CAD build for the part. Positions are in the model's coordinates, mm. A direction names the side the tool comes from. Coordinates: 2 decimals unless noted, no trailing zeros. Write each loop counter-clockwise with the first axis right and the second up, starting at its lowest first coordinate (ties: lowest second). Pieces come first, ordered by that corner, then holes. Notation, with made-up numbers: (-37, -10) -> (-5, -10) arc R7 cw to (-5, 1) -> close; hole circle Ø7 at (38.25, 51). An arc over 180 degrees is marked (long way). Answer as CSV lines item,"result".
```python
from build123d import *

# Parameters (mm, degrees)
DOME1_FACE_RADIUS       = 12.7
DOME1_HEIGHT            = 3.81
CUT_EXTRUDE1_DEPTH      = 53.685870022
CUT_EXTRUDE1_DEPTH_BACK = 53.685870022


with BuildPart() as part:
    # Sketch1 → Revolve2 (revolve)
    with BuildSketch(Plane.XY, mode=Mode.PRIVATE) as revolve2_sk:
        Polygon((0, 0), (0, 45.72), (-12.7, 45.72), (-12.7, 43.18), (-6.35, 43.18), (-6.35, 0), (-0.453180755, 0), align=None)
    revolve(revolve2_sk.sketch.rotate(Axis((0, 0, 0), (0, 1, 0)), 270), axis=Axis((0, 0, 0), (0, 1, 0)))

    # Dome1: a dome of height H over a round flat face of radius A is a cap of a sphere of radius (A * A + H * H) / (2 * H)
    dome1_r = (DOME1_FACE_RADIUS * DOME1_FACE_RADIUS + DOME1_HEIGHT * DOME1_HEIGHT) / (2 * DOME1_HEIGHT)
    dome1_base = Plane((0, 45.72, 0), z_dir=(0, 1, 0))
    with Locations(dome1_base.offset(DOME1_HEIGHT - dome1_r)):
        dome1_ball = Sphere(dome1_r, mode=Mode.PRIVATE)
    add(split(dome1_ball, bisect_by=dome1_base, keep=Keep.TOP, mode=Mode.PRIVATE))

    # Sketch2 → Cut-Extrude1 (cut, two sides: drawn at the far end of the back side and taken through both)
    with BuildSketch(Plane.XY.offset(-CUT_EXTRUDE1_DEPTH_BACK)):
        Polygon((7.09988746, 57.306992364), (-7.09988746, 57.306992364), (-2.413050327, 47.453982482), (2.413050327, 47.453982482), align=None)
    extrude(amount=CUT_EXTRUDE1_DEPTH + CUT_EXTRUDE1_DEPTH_BACK, mode=Mode.SUBTRACT)


solid = part.part
```
Item 1: Saw through at C-C on y = 22. Give the cut face in (x, z).
Answer below:
outline,"circle Ø12.7 at (0, 0)"
Item 2: Saw through at B-B on x = 0. Give the cut face in (y, z).
Answer below:
outline,"(0, -6.35) -> (43.18, -6.35) -> (43.18, -12.7) -> (45.72, -12.7) arc R23.07 ccw to (47.45, -9.56) -> (47.45, 9.56) arc R23.07 ccw to (45.72, 12.7) -> (43.18, 12.7) -> (43.18, 6.35) -> (0, 6.35) -> close"
Item 3: Saw through at A-A on z = 0. Give the cut face in (x, y), and give its area (3 significant figures).
Answer below:
outline,"(-12.7, 43.18) -> (-6.35, 43.18) -> (-6.35, 0) -> (6.35, 0) -> (6.35, 43.18) -> (12.7, 43.18) -> (12.7, 45.72) arc R23.07 ccw to (3.29, 49.29) -> (2.41, 47.45) -> (-2.41, 47.45) -> (-3.29, 49.29) arc R23.07 ccw to (-12.7, 45.72) -> close"
area,"667 mm2"
Item 4: Two-plate mould, pull along X, no slides. Class faces 4 (the flat face through (2.75, 48.16, -0.13)), 5 (the cylindrical face through (7.7, 44.4, 10.1)), 6 (the flat face through (-6, 43.18, -3)): pulls with the +X half, pulls with the -X half, needs draft (parallel to the pull), parting line crosses it, or undercut.
Answer below:
face 4,"undercut"
face 5,"parting line crosses it"
face 6,"needs draft"
Item 5: Saw through at D-D on z = 7.75. Give the cut face in (x, y), and give its area (3 significant figures).
Answer below:
outline,"(-10.06, 43.18) -> (10.06, 43.18) -> (10.06, 45.72) arc R21.73 ccw to (2.68, 48.02) -> (2.41, 47.45) -> (-2.41, 47.45) -> (-2.68, 48.02) arc R21.73 ccw to (-10.06, 45.72) -> close"
area,"81.1 mm2"
Item 6: Wall check: line 1 (Y direction, x = 2.25, z = -8.25); line 2 (Y direction, x = -1.75, z = 5.5); line 3 (X direction, y = 44, z = 0). Give the ranges that are in metal, low to high. Write a range as from..to.
Answer below:
line 1,"y = 43.18..47.45"
line 2,"y = 0..47.45"
line 3,"x = -12.7..12.7"
Item 7: Flat gauge pins, fed straight in: pin 1 (6 mm diameter, centred on x = 9, z = 4.5, fed in from +Y); pin 2 (5.5 mm diameter, centred on x = 0, z = -1, fed in from +Y); pin 3 (12 mm diameter, centred on y = 15.5, z = -9.5, fed in from +X). Where does each tip first touch, or does it go through?
Answer below:
pin 1,"stops at y = 48.42"
pin 2,"stops at y = 48.16"
pin 3,"stops at x = 5.3"
Item 8: 3-axis set-ups, long thin cutter, end or side, ignore diameter. For faces 1 (the cylindrical face through (3.86, 21.29, 5.04)), 2 (the flat face through (-2.76, 48.18, -0.13)), 3 (the flat face through (0, 0, 0)): which of +Z, -Z, +X, -X, +Y, -Y reach the whole face in a straight line?
Answer below:
face 1,"-Y"
face 2,"+Z, -Z, +Y"
face 3,"+Z, -Z, +X, -X, -Y"
